```python
from build123d import *

# Parameters (mm, degrees)
SKETCH2_OUTSIDE_W  = 38.842
SKETCH2_OUTSIDE_H  = 38.842
CUT_EXTRUDE1_DEPTH = 5.8


with BuildPart() as part:
    # Sketch1 → Revolve1 (revolve)
    with BuildSketch(Plane.XY):
        with BuildLine():
            Line((0, 4.1), (0, 5.95))
            Line((0, 5.95), (9.7, 5.95))
            Line((9.7, 5.95), (9.7, 8.5))
            ThreePointArc((9.7, 8.5), (9.992893219, 9.207106781), (10.7, 9.5))
            Line((10.7, 9.5), (27.9, 9.5))
            ThreePointArc((27.9, 9.5), (28.607106781, 9.792893219), (28.9, 10.5))
            Line((28.9, 10.5), (28.9, 12.5))
            Line((28.9, 12.5), (34.7, 12.5))
            Line((34.7, 12.5), (34.7, 9.5))
            ThreePointArc((34.7, 9.5), (34.846446609, 9.146446609), (35.2, 9))
            Line((35.2, 9), (36.7, 9))
            Line((36.7, 9), (36.7, 6.5))
            Line((36.7, 6.5), (36.7, 6))
            ThreePointArc((36.7, 6), (36.846446609, 5.646446609), (37.2, 5.5))
            Line((37.2, 5.5), (39, 5.5))
            ThreePointArc((39, 5.5), (39.353553391, 5.646446609), (39.5, 6))
            Line((39.5, 6), (39.5, 6.5))
            Line((39.5, 6.5), (47.5, 6.5))
            Line((47.5, 6.5), (47.5, 1.6))
            Line((47.5, 1.6), (32.5, 1.6))
            Line((32.5, 1.6), (32.5, 0))
            Line((32.5, 0), (9.4, 0))
            Line((9.4, 0), (9.4, 4.1))
            Line((9.4, 4.1), (0, 4.1))
        make_face()
    revolve(axis=Axis((0, 0, 0), (1, 0, 0)))

    # Sketch2 outside → Cut-Extrude1 (cut)
    with BuildSketch(Plane(origin=(28.9, 0, 0), x_dir=(0, 0, -1), z_dir=(1, 0, 0))):
        Rectangle(SKETCH2_OUTSIDE_W, SKETCH2_OUTSIDE_H)
        Polygon((6.2, 10.854031509), (12.5, 0), (6.2, -10.854031509), (-6.2, -10.854031509), (-12.5, 0), (-6.2, 10.854031509), align=None, mode=Mode.SUBTRACT)
    extrude(amount=CUT_EXTRUDE1_DEPTH, mode=Mode.SUBTRACT)


solid = part.part
```
CAD build for the part. Positions are in the model's coordinates, mm. A direction names the side the tool comes from. Round coordinates to 2 decimals unless told otherwise and drop trailing zeros. Order: outer loops, then holes, each group sorted by start corner. A loop starts at its lowest first (then second) coordinate and runs counter-clockwise, first axis right, second up. Notation, with made-up numbers: (15.5, 89.25) -> (70.5, 89.25) arc R16 ccw to (70.5, 102.25) -> close; hole circle Ø8 at (5.5, 36.25). An arc over 180 degrees is marked (long way). One line per question, with ' | ' between items.
Q1. Slice it at B-B (x = 24). Write the cut outline in (y, z).
Completed:
outline: circle Ø19 at (0, 0)
Q2. Which spindle directions (+Z, -Z, +X, -X, +Y, -Y) get a long thin tool onto all of the face, cutting with end or side? Do faces 1 (the flat face through (39.5, -2, -6)), 2 (the cylindrical face through (4.918, -4.385, 4.021)), 3 (the flat face through (31.759, 5.351, 9.394)), 4 (the flat face through (34.7, 3.2, -9.2)). Say none if no direction does.
Completed:
face 1: none | face 2: -X | face 3: +Z, +X, -X, +Y | face 4: +X
Q3. Slice it at C-C (x = 38). Write the cut outline in (y, z).
Completed:
outline: circle Ø11 at (0, 0); hole circle Ø3.2 at (0, 0)
Q4. Two-plate mould, pull along Y, no slides. Class faces 5 (the flat face through (9.4, 0, 0)), 6 (the cylindrical face through (43.556, -5.158, -3.955)), 7 (the flat face through (31.759, -5.503, 9.306)): released by +Y, released by -Y, zero draft, split by the parting line, or undercut.
Completed:
face 5: undercut | face 6: split by the parting line | face 7: released by -Y
Q5. Drop flat-ended pins along their axis: pin 1 (4 mm diameter, centred on x = 16.5, z = 2.5, fed in from +Y); pin 2 (6 mm diameter, centred on x = 14.5, y = 1.5, fed in from +Z); pin 3 (3 mm diameter, centred on y = 0, z = 0, fed in from -X). Give the stop position or say it passes through.
Completed:
pin 1: stops at y = 9.49 | pin 2: stops at z = 9.5 | pin 3: stops at x = 9.4
Q6. Slice it at A-A (x = 33). Write the cut outline in (y, z), then the cut area to 3 significant figures.
Completed:
outline: (-10.85, -6.2) -> (0, -12.5) -> (10.85, -6.2) -> (10.85, 6.2) -> (0, 12.5) -> (-10.85, 6.2) -> close; hole circle Ø3.2 at (0, 0) | area: 398 mm^2
Q7. Probe probe 1 along Z at (x, y) = (5, 0); probe 2 along Z at (x, y) = (41.25, 0); probe 3 along X at (y, z) = (4.75, -5). List the from-to ranges inside material, lowest first.
Completed:
probe 1: z = -5.95 to -4.1, 4.1 to 5.95 | probe 2: z = -6.5 to -1.6, 1.6 to 6.5 | probe 3: x = 9.7 to 36.7
